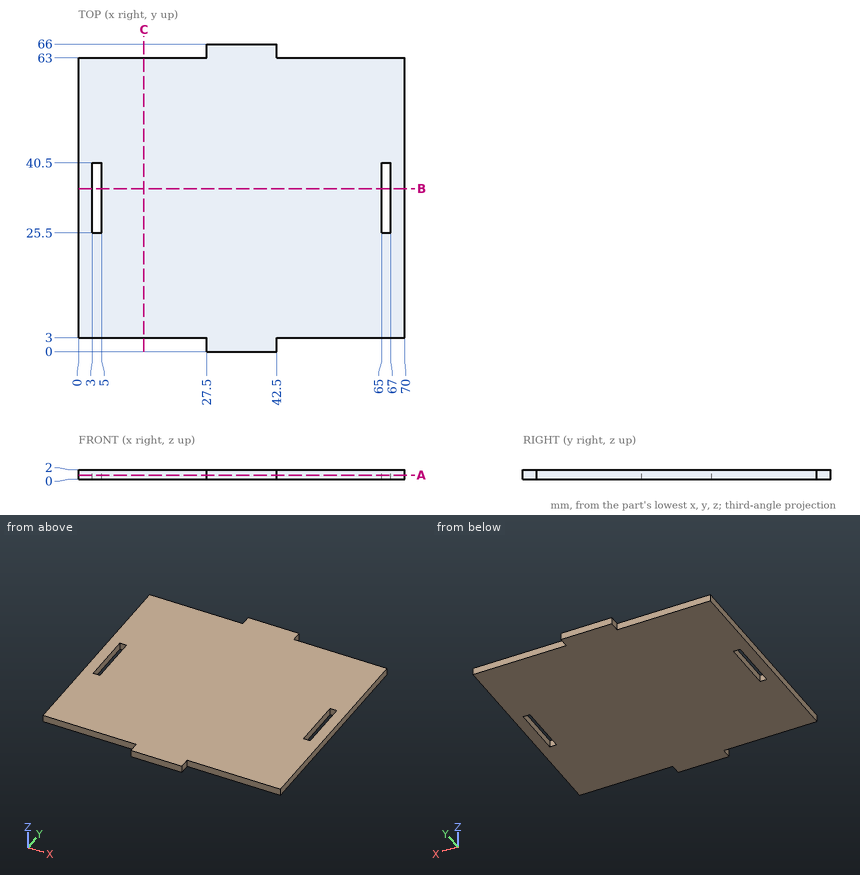
Geometry: see drawing. Coordinates: mm, zero at the bounding-box minimum. Give positions to 0.01 mm unless a question says otherwise; leave off trailing zeros. Loops run counter-clockwise (first coordinate to the right, second up) from the corner with the lowest first, then second, coordinate; pieces in that order, holes last. Notation, with made-up numbers: (-32.75, 55.25) - (12.25, 55.25) arc R26 cw to (12.25, 77.25) - close; hole circle Ø8 at (51.25, 89). An arc over 180 degrees is marked (long way). Use CSV: the item, a comma, the result in double quotes. Start each with the question number.
1. Section C-C (x = 14). Output: boundary loops of the cut face in (y, z), then the cut area to 3 significant figures.
2. Section B-B (y = 35). Output: boundary loops of the cut face in (x, z).
3. Ray query, L1, parallel to X at y = 32, z = 0.8; L2, parallel to Y at x = 66.5, z = 0.2; L3, parallel to Y at x = 12, z = 1.4. Return the intervals inside material, ascending.
4. Section A-A (z = 0.85). Output: boundary loops of the cut face in (x, y), then the cut area to 3 significant figures.
5. Pin query (flat end, axial travel): pin 1 (0.6 mm diameter, centred on x = 10, z = 1, fed in from +Y); pin 2 (0.6 mm diameter, centred on x = 4.5, z = 1, fed in from -Y); pin 3 (1 mm diameter, centred on y = 2, z = 1, fed in from -X). Return the tip coordinate at first contact, or that it passes through.
Response:
1,outline,"(3, 0) - (63, 0) - (63, 2) - (3, 2) - close"
1,area,"120 mm²"
2,outline,"(0, 0) - (3, 0) - (3, 2) - (0, 2) - close; (5, 0) - (65, 0) - (65, 2) - (5, 2) - close; (67, 0) - (70, 0) - (70, 2) - (67, 2) - close"
3,L1,"0 to 3, 5 to 65, 67 to 70"
3,L2,"3 to 25.5, 40.5 to 63"
3,L3,"3 to 63"
4,outline,"(0, 3) - (27.5, 3) - (27.5, 0) - (42.5, 0) - (42.5, 3) - (70, 3) - (70, 63) - (42.5, 63) - (42.5, 66) - (27.5, 66) - (27.5, 63) - (0, 63) - close; hole (3, 25.5) - (5, 25.5) - (5, 40.5) - (3, 40.5) - close; hole (65, 25.5) - (67, 25.5) - (67, 40.5) - (65, 40.5) - close"
4,area,"4,230 mm²"
5,pin 1,"y = 63"
5,pin 2,"y = 3"
5,pin 3,"x = 27.5"
